Part model, mm, in its own coordinate system. A direction names the side the tool comes from. Round coordinates to 2 decimals unless told otherwise and drop trailing zeros. Loops run counter-clockwise (first coordinate to the right, second up) from the corner with the lowest first, then second, coordinate; pieces in that order, holes last.
1) Band-saw the part on D-D, the plane y = 8. Write the cut outline in (x, z).
2) Band-saw the part on A-A, the plane x = 0. Write the cut outline in (y, z), then the cut area to 3 significant figures.
3) Mould opens along Y. For faces 3 (the flat face through (0, -7, 17.78)), 4 (the flat face through (0, 5.955, 9)), 5 (the cylindrical face through (-3.772, -16.985, 8.766)) say: +Y half, -Y half, draft (parallel to the pull), parting line (faces both ways), or undercut.
4) Band-saw the part on B-B, the plane y = 0. Write the cut outline in (x, z), then the cut area to 3 significant figures.
5) Band-saw the part on C-C, the plane z = 16.25. Write the cut outline in (x, y).
6) Probe line 1 (X direction, y = 5.5, z = 14.5); line 2 (Y direction, x = -6, z = 1.25); line 3 (Y direction, x = 3, z = 4.75). List the from-to ranges inside material, lowest first.
7) Drop flat-ended pins along their axis: P1, Ø4, axis at y = 9, z = 15, coming from the -X side; P2, Ø3, axis at x = -3, z = 2.5, coming from the +Y side; P3, Ø6, axis at x = -10.5, z = 12.5, coming from the +Y side. Give the stop position or say it passes through.
8) 3-axis set-ups, long thin cutter, end or side, ignore diameter. For faces 1 (the flat face through (0, -7, 0)), 2 (the cylindrical face through (-3.23, 5.62, 9.01)): which of +Z, -Z, +X, -X, +Y, -Y reach the whole face in a straight line?
from build123d import *

# Parameters (mm, degrees)
SKETCH1_R           = 17.399
BOSS_EXTRUDE1_DEPTH = 17.78
FILLET1_R           = 2.54


with BuildPart() as part:
    # Sketch1 → Boss-Extrude1 (new body)
    with BuildSketch(Plane.XY):
        Circle(SKETCH1_R)
        Polygon((6.87578, 0), (3.43789, 5.954600151), (-3.43789, 5.954600151), (-6.87578, 0), (-3.43789, -5.954600151), (3.43789, -5.954600151), align=None, mode=Mode.SUBTRACT)
    extrude(amount=BOSS_EXTRUDE1_DEPTH)

    # Fillet1
    fillet1_edges = [part.edges().sort_by_distance(p)[0] for p in [
        (6.87578, 0, 8.89),
        (3.43789, 5.954600151, 8.89),
        (-3.43789, 5.954600151, 8.89),
        (-6.87578, 0, 8.89),
        (-3.43789, -5.954600151, 8.89),
        (3.43789, -5.954600151, 8.89),
    ]]
    fillet(fillet1_edges, radius=FILLET1_R)


solid = part.part
Reported:
1. outline: (-15.45, 0) - (15.45, 0) - (15.45, 17.78) - (-15.45, 17.78) - close
2. outline: (-17.4, 0) - (-5.95, 0) - (-5.95, 17.78) - (-17.4, 17.78) - close; (5.95, 0) - (17.4, 0) - (17.4, 17.78) - (5.95, 17.78) - close
2. area: 407 mm2
3. face 3: draft
3. face 4: undercut
3. face 5: parting line
4. outline: (-17.4, 0) - (-6.48, 0) - (-6.48, 17.78) - (-17.4, 17.78) - close; (6.48, 0) - (17.4, 0) - (17.4, 17.78) - (6.48, 17.78) - close
4. area: 388 mm2
5. outline: circle Ø34.8 at (0, 0); hole (-6.14, -1.27) - (-4.17, -4.68) arc R2.54 ccw to (-1.97, -5.95) - (1.97, -5.95) arc R2.54 ccw to (4.17, -4.68) - (6.14, -1.27) arc R2.54 ccw to (6.14, 1.27) - (4.17, 4.68) arc R2.54 ccw to (1.97, 5.95) - (-1.97, 5.95) arc R2.54 ccw to (-4.17, 4.68) - (-6.14, 1.27) arc R2.54 ccw to start
6. line 1: x = -16.51 to -3.42, 3.42 to 16.51
6. line 2: y = -16.33 to -1.52, 1.52 to 16.33
6. line 3: y = -17.14 to -5.74, 5.74 to 17.14
7. P1: stops at x = -15.93
7. P2: stops at y = 17.33
7. P3: stops at y = 15.7
8. face 1: -Z, +X, -X, +Y, -Y
8. face 2: +Z, -Z
